Autodesk Inventor part; units mm, degrees
ref_plane "YZ Plane" through (0, 0, 0) normal (1, 0, 0) x (0, 1, 0)
ref_plane "XZ Plane" through (0, 0, 0) normal (0, 1, 0) x (-1, 0, 0)
ref_plane "XY Plane" through (0, 0, 0) normal (0, 0, 1) x (1, 0, 0)
sketch "スケッチ1" plane through (0, 0, 0) normal (0, 1, 0) x (-1, 0, 0)
  line L0 (0, 0) -> (0, -43)
  line L1 (0, -43) -> (32, -43)
  line L2 (32, -43) -> (32, 0)
  line L3 (32, 0) -> (0, 0)
  dimension "d0" = 43
  dimension "d1" = 32
extrude "押し出し1" add sketch "スケッチ1" along normal blind 39.5
fillet "フィレット1" radius 2 2 edges at (-32, 19.75, 0) (0, 19.75, 0)
sketch "スケッチ2" plane through (0, 39.5, 0) normal (0, 1, 0) x (1, 0, 0)
  line L0 (0, 43) -> (-32, 43)
  line L1 (-16, 43) -> (-16, 0)
  line L2 (-30, 0) -> (-2, 0)
  line L3 (-16, 21.5) -> (-16, 3)
  line L4 (-16, 3) -> (-2.5, 3)
  line L5 (0, 2) -> (0, 43)
  line L6 (-16, 3) -> (-29.5, 3)
  line L7 (-29.5, 3) -> (-29.5, 30)
  point P0 (0, 0)
  point P1 (-2.5, 30)
  dimension "d5" = 18.5
  dimension "d6" = 13.5
  dimension "d7" = 13.5
  dimension "d8" = 27
hole "穴1" at (-2.5, 39.5, -3) at (-29.5, 39.5, -3) at (-29.5, 39.5, -30) at (-2.5, 39.5, -30) direction (0, -1, 0) diameter 2.6 end through all
sketch "スケッチ3" plane through (0, 39.5, 0) normal (0, 1, 0) x (1, 0, 0)
  line L0 (0, 43) -> (-32, 43)
  line L1 (-16, 43) -> (-16, 0)
  line L2 (-16, 21.5) -> (-16, 31)
  line L3 (-32, 43) -> (-32, 2)
  line L4 (-32, 31) -> (-32, 43)
  line L5 (-32, 43) -> (-26.583, 43)
  line L6 (0, 2) -> (0, 43)
  line L7 (0, 31) -> (0, 43)
  line L8 (0, 43) -> (-5.417, 43)
  arc A0 (-26.583, 43) -> (-32, 31) centre (-16, 31) ccw
  arc A1 (0, 31) -> (-5.417, 43) centre (-16, 31) ccw
  point P0 (0, 0)
  dimension "d16" = 9.5
extrude "押し出し2" cut sketch "スケッチ3" against normal blind 39.5
sketch "スケッチ4" plane through (0, 39.5, 0) normal (0, 1, 0) x (1, 0, 0)
  arc A0 (-26.583, 43) -> (-32, 31) centre (-16, 31) ccw
  circle A1 centre (-16, 31) radius 4
  point P0 (0, 0)
  dimension "d20" = 8
extrude "押し出し3" add sketch "スケッチ4" along normal blind 5
sketch "スケッチ5" plane through (0, 0, 0) normal (0, -1, 0) x (1, 0, 0)
  circle A0 centre (-16, -31) radius 4
  circle A1 centre (-16, -31) radius 4
  point P0 (0, 0)
extrude "押し出し4" add sketch "スケッチ5" along normal blind 5.5
sketch "スケッチ6" plane through (0, 0, 0) normal (0, -1, 0) x (1, 0, 0)
  line L0 (-30, 0) -> (-2, 0)
  line L1 (-16, 0) -> (-1.6, 0)
  line L2 (-1.6, 0) -> (-1.6, 8.5)
  line L3 (-1.6, 0) -> (6.9, 0) construction
  line L4 (-1.6, 8.5) -> (-30.4, 8.5)
  line L5 (-30.4, 8.5) -> (-30.4, -0.1236)
  line L6 (-30.4, -0.1236) -> (-1.6, -0.1236)
  line L7 (-1.6, -0.1236) -> (-1.6, 0)
  point P0 (0, 0)
  dimension "d25" = 14.4
  dimension "d26" = 8.5
  dimension "d27" = 90
  dimension "d28" = 28.8
extrude "押し出し5" add sketch "スケッチ6" against normal blind 11.8
sketch "スケッチ7" plane through (0, 0, 0) normal (0, -1, 0) x (1, 0, 0)
  arc A0 (0, -2) -> (-2, 0) centre (-2, -2) ccw
  arc A1 (-1.6, -0.0404) -> (-2, 0) centre (-2, -2) ccw
  arc A2 (-30.4, -0.0404) -> (-32, -2) centre (-30, -2) ccw
  arc A3 (-30, 0) -> (-30.4, -0.0404) centre (-30, -2) ccw
  line L0 (-1.6, -0.0404) -> (-1.6, 8.5)
  line L1 (-1.6, 8.5) -> (-30.4, 8.5)
  line L2 (-30.4, 8.5) -> (-1.6, 8.5)
  line L3 (-30.4, 8.5) -> (-30.4, -0.0404)
  line L4 (-30, 0) -> (-2, 0)
  arc A4 (-30, 0) -> (-30.4, -0.0404) centre (-30, -2) ccw
  point P0 (0, 0)
extrude "押し出し6" cut sketch "スケッチ7" against normal blind 0.2
thread "ねじ1"
thread "ねじ2"
thread "ねじ3"
thread "ねじ4"
sketch "スケッチ12" plane through (-16, 45, -31) normal (0, 1, 0) x (1, 0, 0)
  circle A0 centre (0, 0) radius 10.5
  point P0 (16, -31)
  dimension "d66" = 21
extrude "押し出し9" add sketch "スケッチ12" against normal blind 5
sketch "スケッチ13" plane through (-16, 45, -31) normal (0, 1, 0) x (1, 0, 0)
  circle A0 centre (0, 0) radius 5
  point P0 (16, -31)
  dimension "d69" = 10
extrude "押し出し10" add sketch "スケッチ13" along normal blind 1
sketch "スケッチ14" plane through (-16, 45, -31) normal (0, 1, 0) x (1, 0, 0)
  circle A0 centre (0, 0) radius 8.5
  circle A1 centre (0, 8.5) radius 1.3
  circle A2 centre (-8.5, 0) radius 1.3
  circle A3 centre (8.5, 0) radius 1.3
  circle A4 centre (0, -8.5) radius 1.3
  point P0 (16, -31)
  dimension "d72" = 17
  dimension "d73" = 2.6
  dimension "d74" = 2.6
  dimension "d75" = 2.6
  dimension "d76" = 2.6
extrude "押し出し11" cut sketch "スケッチ14" against normal blind 5 contours A0 A3 | A0 A3 | A1 A0 | A0 A1 | A4 A0 | A0 A4 | A2 A0 | A0 A2
thread "ねじ9"
thread "ねじ10"
thread "ねじ11"
thread "ねじ12"
sketch "スケッチ15" plane through (0, 0, 0) normal (0, -1, 0) x (1, 0, 0)
  circle A0 centre (-16, -31) radius 4
  circle A1 centre (-16, -31) radius 6
  point P0 (0, 0)
  dimension "d87" = 12
extrude "押し出し12" add sketch "スケッチ15" along normal blind 1.8
sketch "スケッチ16" plane through (-16, -5.5, -31) normal (0, -1, 0) x (1, 0, 0)
  point P0 (16, 31)
  point P1 (0, 0)
hole "穴3" at (-16, -5.5, -31) direction (0, 1, 0) diameter 3 depth 8 tip angle 118
thread "ねじ13"
properties part number "B3M11xx" material "アルミニウム 2014-T4"
Geometry check sheet. Reference: the model listing, model coordinates, mm. A direction names the side the tool comes from. Round coordinates to 2 decimals unless told otherwise and drop trailing zeros. Order: outer loops, then holes, each group sorted by start corner. A loop starts at its lowest first (then second) coordinate and runs counter-clockwise, first axis right, second up. Notation, with made-up numbers: M 56,-40 L 97,-40 A38 ccw 97,-1 Z; hole C -27.75,85 d8. An arc over 180 degrees is marked long. Answer in a Markdown table with one row per item. Add a question column.
Item 1: Sectioned sample at B-B, the plane y = 6. Enter the section's corners in (x, z).
Item 2: Sectioned sample at A-A, the plane z = -3. Enter the section's corners in (x, y).
Item 3: Set-up check for faces 1 (the face through (-11, 40, -31)), 2 (the face through (-17.03, 42.54, -21.71)), 3 (the face through (-16, 11.8, 4)), 4 (the face through (-1.6, 6, 4)): record each of +Z, -Z, +X, -X, +Y, -Y from which the full face is reachable in a straight line by a thin tool's end or side.
Item 4: Depth check by flat-ended pin: pin 1 Ø3 at (x, z) = (-16, -22.5) entering from -Y; pin 2 Ø1.6 at (x, z) = (-16, -39.5) entering from +Y; pin 3 Ø2.5 at (x, z) = (-17.5, 4.5) entering from +Y. Enter the tip coordinate at first touch or a pass-through.
Item 5: Sectioned sample at C-C, the plane x = -19. Enter the section's corners in (y, z).
Item 6: Sectioned sample at D-D, the plane y = 19. Enter the section's corners in (x, z), plus the area to 3 significant figures.
Item 7: Draft check along Z on faces 5 (the face through (-25.458, 42.535, -31.879)), 6 (the face through (-17.301, -0.887, -25.143)), 7 (the face through (-16, 39.5, -21)), 8 (the face through (-30.544, 20.026, -37.669)). Enter one of: released by +Z, released by -Z, zero draft, split by the parting line, or undercut.
Item 8: Material ranges on L1, parallel to X at y = 42, z = -31; L2, parallel to Z at x = -16, y = 41.25; L3, parallel to Z at x = -29, y = 20, recorded low to high. Write a range as [from, to].
Filled in:
| question | item | result |
|---|---|---|
| 1 | outline | M -32,-31 A16 ccw -26.58,-43 L -5.42,-43 A16 ccw 0,-31 L 0,-2 A2 ccw -1.6,-0.04 L -1.6,8.5 L -30.4,8.5 L -30.4,-0.04 A2 ccw -32,-2 Z; hole C -29.5,-30 d2.6; hole C -29.5,-3 d2.6; hole C -2.5,-30 d2.6; hole C -2.5,-3 d2.6 |
| 2 | outline | M -32,0 L -30.8,0 L -30.8,39.5 L -32,39.5 Z; M -28.2,0 L -3.8,0 L -3.8,39.5 L -28.2,39.5 Z; M -1.2,0 L 0,0 L 0,39.5 L -1.2,39.5 Z |
| 3 | face 1 | none |
| 3 | face 2 | +Y |
| 3 | face 3 | +Z, +X, -X, +Y |
| 3 | face 4 | +Z, +X, +Y, -Y |
| 4 | pin 1 | stops at y = 0 |
| 4 | pin 2 | stops at y = 39.5 |
| 4 | pin 3 | stops at y = 11.8 |
| 5 | outline | M -5.5,-33.65 L -1.8,-33.65 L -1.8,-36.2 L 0,-36.2 L 0,-43 L 39.5,-43 L 39.5,-33.65 L 40,-33.65 L 40,-41.06 L 45,-41.06 L 45,-35 L 46,-35 L 46,-27 L 45,-27 L 45,-20.94 L 40,-20.94 L 40,-28.35 L 39.5,-28.35 L 39.5,0 L 11.8,0 L 11.8,8.5 L 0.2,8.5 L 0.2,0 L 0,0 L 0,-25.8 L -1.8,-25.8 L -1.8,-28.35 L -5.5,-28.35 Z |
| 6 | outline | M -32,-31 A16 ccw -26.58,-43 L -5.42,-43 A16 ccw 0,-31 L 0,-2 A2 ccw -2,0 L -30,0 A2 ccw -32,-2 Z; hole C -29.5,-30 d2.6; hole C -29.5,-3 d2.6; hole C -2.5,-30 d2.6; hole C -2.5,-3 d2.6 |
| 6 | area | 1,310 mm² |
| 7 | face 5 | undercut |
| 7 | face 6 | split by the parting line |
| 7 | face 7 | zero draft |
| 7 | face 8 | released by -Z |
| 8 | L1 | x = [-26.5, -25.8], [-23.2, -8.8], [-6.2, -5.5] |
| 8 | L2 | z = [-41.5, -40.8], [-38.2, -23.8], [-21.2, -20.5] |
| 8 | L3 | z = [-40.33, -31.2], [-28.8, -4.2], [-1.8, 0] |
